Model file for the job. Use its own axes, mm. A direction names the side the tool comes from. Coordinates: 2 decimals unless noted, no trailing zeros. Write each loop counter-clockwise with the first axis right and the second up, starting at its lowest first coordinate (ties: lowest second). Pieces come first, ordered by that corner, then holes. Notation, with made-up numbers: (45, -6) - (84, -6) arc R13 ccw to (84, 18) - close; hole circle Ø7 at (59, -19.75). An arc over 180 degrees is marked (long way). Put each result on its own line as item: value. Start each with the question number.
1. Saw through at B-B, the plane x = -4.5. Write the cut outline in (y, z).
2. Drill centre lines: L1, parallel to X at y = 0, z = 8; L2, parallel to X at y = -0.75, z = 7; L3, parallel to X at y = 9.25, z = 17.25. Where is each one in solid material? Low to high. Write a range as from..to.
3. Saw through at C-C, the plane z = 2.75. Write the cut outline in (x, y), plus the area to 3 significant figures.
4. Pull direction X, two halves, no side cores. Call faces 5 (the face through (-1, 11, 19.9)), 6 (the face through (15.17, -3.06, 9.81)): released by +X, released by -X, zero draft, split by the parting line, or undercut.
5. Saw through at A-A, the plane y = -2.25. Write the cut outline in (x, z), plus the area to 3 significant figures.
6. Drop flat-ended pins along their axis: P1, Ø6, axis at x = -9.5, z = 5, coming from the +Y side; P2, Ø1.5, axis at x = 9, y = 2.5, coming from the -Z side; P3, Ø9.5, axis at y = 7, z = 9, coming from the +X side. Give the stop position or say it passes through.
7. Which spindle directions (+Z, -Z, +X, -X, +Y, -Y) get a long thin tool onto all of the face, cutting with end or side? Do faces 1 (the face through (13.9, -1.5, 9.8)), 2 (the face through (9.386, 4, 15)), 3 (the face through (-10.4, 2.7, 1.6)), 4 (the face through (13, 3, 10)). Say none if no direction does.
8. Saw through at D-D, the plane x = 8. Write the cut outline in (y, z).
```python
from build123d import *

# Parameters (mm, degrees)
F0_R      = 3.75
F0_R_2    = 1.75
F1_DEPTH  = 19.9
F2_W      = 18.7715838526
F2_H      = 2
F5_W      = 18.7715838526
F5_H      = 2
F8_R      = 5.25
F9_DEPTH  = 11.6830509442
F11_DEPTH = 2
F12_W     = 1.6142080737
F12_H     = 6.9905174896
F13_DEPTH = 19.9010001


# Not quite as in the source:
# - a pattern or mirror of a feature is missing from the dataset's text; its kind, count and spacing are read off the source's solid


with BuildPart() as f1:
    # F0 (on Top) → F1 (new body)
    with BuildSketch(Plane.XY):
        with Locations((13, 0)):
            Circle(F0_R)
        with Locations((13, 0)):
            Circle(F0_R_2, mode=Mode.SUBTRACT)
    extrude(amount=F1_DEPTH)



with BuildPart() as f1b:
    # F0 (on Top) → F1, piece 2 (new body)
    with BuildSketch(Plane.XY):
        with Locations((-13, 0)):
            Circle(F0_R)
        with Locations((-13, 0)):
            Circle(F0_R_2, mode=Mode.SUBTRACT)
    extrude(amount=F1_DEPTH)


with BuildPart() as f1_1:
    add(f1.part)

    add(f1b.part)  # F6 merges F1b
    # F2 (on Top) → F6 section 0
    with BuildSketch(Plane.XY):
        Rectangle(F2_W, F2_H)
    # F5 (on offset) → F6 section 1
    with BuildSketch(Plane.XY.offset(19.9)):
        with Locations((0, 11.4892703569)):
            Rectangle(F5_W, F5_H)
    loft()

    # F8 (on offset) → F9 (cut, through all)
    with BuildSketch(Plane(origin=(0, -0.75, 0.4330127019), x_dir=(1, 0, 0), z_dir=(0, -0.8660254038, 0.5))):
        with Locations((0, 10.9892703569)):
            Circle(F8_R)
    extrude(amount=-F9_DEPTH, mode=Mode.SUBTRACT)

    # F10 (on face) → F11 (join)
    with BuildSketch(Plane(origin=(-9.3857919263, 0, 0), x_dir=(0, -1, 0), z_dir=(-1, 0, 0))):
        Polygon((-1, 19.9), (-12.4892703569, 19.9), (-1, 0), (-1, 3.4641016151), align=None)
    f11 = extrude(amount=F11_DEPTH)

    # F11_copies: F11 across plane
    add(f11.mirror(Plane(origin=(0, 0, 0), x_dir=(0, 0, 1), z_dir=(1, 0, 0))))

    # F12 (on Top) → F13 (cut, through all)
    with BuildSketch(Plane.XY):
        with Locations((-12.1928959631, 3.4952587448)):
            Rectangle(F12_W, F12_H)
    f13 = extrude(amount=F13_DEPTH, mode=Mode.SUBTRACT)

    # F13_copies: F13 across plane
    add(f13.mirror(Plane(origin=(0, 0, 0), x_dir=(0, 0, 1), z_dir=(1, 0, 0))), mode=Mode.SUBTRACT)


solid = f1_1.part
```
Final values:
1. outline: (-1, 0) - (1, 0) - (4.89, 6.74) - (3.39, 7.61) - close; (6.1, 12.29) - (7.6, 11.43) - (12.49, 19.9) - (10.49, 19.9) - close
2. L1: x = -16.75..-14.75, -11.25..-9.25, 9.25..11.25, 14.75..16.75
2. L2: x = -16.67..-14.58, -11.42..-9.33, 9.33..11.42, 14.58..16.67
2. L3: x = -11.39..11.39
3. outline: (-13, 1.75) - (-13, 3.75) arc R3.75 ccw (long way) to (-9.3, 0.59) - (9.3, 0.59) arc R3.75 ccw (long way) to (13, 3.75) - (13, 1.75) arc R1.75 cw (long way) to (11.39, 0.68) - (11.39, 3.38) arc R3.75 ccw to (10.29, 2.59) - (-10.29, 2.59) arc R3.75 ccw to (-11.39, 3.38) - (-11.39, 0.68) arc R1.75 cw (long way) to start
3. area: 101 mm²
4. face 5: zero draft
4. face 6: undercut
5. outline: (-16, 0) - (-10, 0) - (-10, 19.9) - (-16, 19.9) - close; (10, 0) - (16, 0) - (16, 19.9) - (10, 19.9) - close
5. area: 239 mm²
6. P1: stops at y = 5.62
6. P2: stops at z = 1.3
6. P3: stops at x = 16
7. face 1: +Z, -Z
7. face 2: +Z
7. face 3: -Z, +Y
7. face 4: +Z, -Z, +Y
8. outline: (-1, 0) - (1, 0) - (12.49, 19.9) - (10.49, 19.9) - close
